Input: part model. Units: mm. Frame: model coordinates. Round coordinates to 2 decimals unless told otherwise and drop trailing zeros.
Item 1: Line query: L1, parallel to Y at x = 22.6, z = 0.95; L2, parallel to Y at x = 130.9, z = 0.9; L3, parallel to Y at x = 137, z = 0.8. Output: solid intervals per line, ascending.
Item 2: Cut plane A-A on z = 1.55. Give the number of separate pieces and of enclosed holes in the cut face, then the cut area to 3 significant figures.
Item 3: First-contact query: pin 1 (0.7 mm diameter, centred on x = -65, z = 1.5, fed in from -Y); pin 2 (1.1 mm diameter, centred on x = 15.5, z = 1, fed in from +Y); pin 3 (11 mm diameter, centred on x = -7.88, y = -1.6, fed in from +Z). Flat tips, straight axial feed; report the tip coordinate or a pass-through.
```python
from build123d import *

# Parameters (mm, degrees)
F0_R     = 1.9
F0_R_2   = 8.05
F0_R_3   = 1.475
F0_W     = 24.5
F0_H     = 14.25
F3_DEPTH = 2.286
F2_R     = 1.75
F2_W     = 90
F2_H     = 34
F4_DEPTH = 2.286
F1_R     = 1.55
F1_R_2   = 1.9
F1_R_3   = 1.75
F1_R_4   = 6.72
F1_W     = 6.5
F1_H     = 3
F5_DEPTH = 2.286


with BuildPart() as f3:
    # F0 (on Top) → F3 (new body)
    with BuildSketch(Plane.XY):
        with BuildLine():
            Line((-17.961566, 79.945827), (-158.734, 79.945827))
            ThreePointArc((-158.734, 79.945827), (-172.922805, 74.068631), (-178.8, 59.879827))
            Line((-178.8, 59.879827), (-178.8, -61.988173))
            ThreePointArc((-178.8, -61.988173), (-172.922805, -76.176978), (-158.734, -82.054173))
            Line((-158.734, -82.054173), (-79.8, -82.054173))
            Line((-79.8, -82.054173), (-72.08434, -79.454173))
            Line((-72.08434, -79.454173), (-62.08434, -79.454173))
            Line((-62.08434, -79.454173), (-54.3, -82.054173))
            Line((-54.3, -82.054173), (54.3, -82.054173))
            Line((54.3, -82.054173), (62.084, -79.454173))
            Line((62.084, -79.454173), (72.084, -79.454173))
            Line((72.084, -79.454173), (79.8, -82.054173))
            Line((79.8, -82.054173), (158.734, -82.054173))
            ThreePointArc((158.734, -82.054173), (172.922805, -76.176978), (178.8, -61.988173))
            Line((178.8, -61.988173), (178.8, 59.879827))
            ThreePointArc((178.8, 59.879827), (172.922805, 74.068631), (158.734, 79.945827))
            Line((158.734, 79.945827), (17.961566, 79.945827))
            Line((17.961566, 79.945827), (6.5, 77.595827))
            Line((6.5, 77.595827), (-6.5, 77.595827))
            Line((-6.5, 77.595827), (-17.961566, 79.945827))
        make_face()
        with Locations((-130.9, -69.243173)):
            Circle(F0_R, mode=Mode.SUBTRACT)
        with Locations((-165.989, -40.1)):
            Circle(F0_R, mode=Mode.SUBTRACT)
        with Locations((130.9, -69.243173)):
            Circle(F0_R, mode=Mode.SUBTRACT)
        with Locations((165.989, -40.1)):
            Circle(F0_R, mode=Mode.SUBTRACT)
        with Locations((-165.989, 36.1)):
            Circle(F0_R, mode=Mode.SUBTRACT)
        with Locations((-128.8, 39.945827)):
            Circle(F0_R_2, mode=Mode.SUBTRACT)
        with Locations((-130.9, 67.134827)):
            Circle(F0_R, mode=Mode.SUBTRACT)
        with Locations((165.989, 36.1)):
            Circle(F0_R, mode=Mode.SUBTRACT)
        with Locations((113.525, 39.945827)):
            Circle(F0_R_3, mode=Mode.SUBTRACT)
        with Locations((128.8, 39.945827)):
            Rectangle(F0_W, F0_H, mode=Mode.SUBTRACT)
        with Locations((144.075, 39.95638)):
            Circle(F0_R_3, mode=Mode.SUBTRACT)
        with Locations((130.9, 67.134827)):
            Circle(F0_R, mode=Mode.SUBTRACT)
    extrude(amount=F3_DEPTH)

    # F2 (on face) → F4 (cut)
    with BuildSketch(Plane.XY):
        with Locations((-143.8, 12.895827)):
            Circle(F2_R)
        with Locations((-143.8, -42.054173)):
            Circle(F2_R)
        with Locations((-50.75, 12.895827)):
            Circle(F2_R)
        with Locations((-50.75, -42.054173)):
            Circle(F2_R)
        with Locations((-97.275, -14.579173)):
            Rectangle(F2_W, F2_H)
    extrude(amount=F4_DEPTH, mode=Mode.SUBTRACT)

    # F1 (on face) → F5 (cut)
    with BuildSketch(Plane.XY):
        with Locations((96.275749, -42.242036)):
            Circle(F1_R)
        with Locations((96.275749, 44.117964)):
            Circle(F1_R)
        with Locations((-28.2, 44.117964)):
            Circle(F1_R)
        with Locations((-28.2, -42.242036)):
            Circle(F1_R)
        with Locations((-26.94, -32.082036)):
            Circle(F1_R_2)
        with Locations((22.6, -27.002036)):
            Circle(F1_R_3)
        with Locations((-23.12, -16.842036)):
            Circle(F1_R_4)
        with Locations((-7.88, -16.842036)):
            Circle(F1_R_4)
        with Locations((-7.88, -1.602036)):
            Circle(F1_R_4)
        with Locations((7.36, -16.842036)):
            Circle(F1_R_4)
        with Locations((-7.88, -32.082036)):
            Circle(F1_R_4)
        with Locations((-12.49, 44.157964)):
            Rectangle(F1_W, F1_H)
        with Locations((-3.365, 44.157964)):
            Rectangle(F1_W, F1_H)
        with Locations((5.76, 44.157964)):
            Rectangle(F1_W, F1_H)
        with Locations((14.885, 44.157964)):
            Rectangle(F1_W, F1_H)
        with Locations((24.01, 44.157964)):
            Rectangle(F1_W, F1_H)
    extrude(amount=F5_DEPTH, mode=Mode.SUBTRACT)


solid = f3.part
```
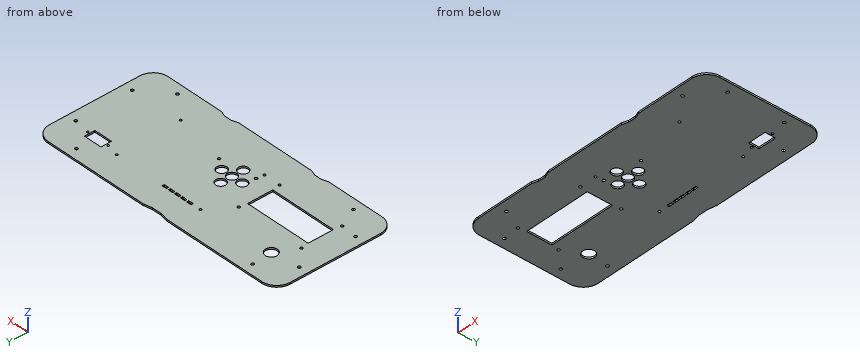
From the geometry:
1. L1: y = -82.05 to -28.75, -25.25 to 42.66, 45.66 to 79.95
1. L2: y = -82.05 to -71.14, -67.34 to 32.82, 47.07 to 65.23, 69.03 to 79.95
1. L3: y = -82.05 to 32.82, 47.07 to 79.95
2. separate pieces: 1
2. enclosed holes: 33
2. area: 52,800 mm2
3. pin 1: stops at y = -79.45
3. pin 2: stops at y = 79.55
3. pin 3: passes through
